Drawing for the job (mm, zero at the part's lowest x, y, z). A direction names the side the tool comes from. Round coordinates to 2 decimals unless told otherwise and drop trailing zeros. Write each loop counter-clockwise with the first axis right and the second up, starting at its lowest first coordinate (ties: lowest second). Pieces come first, ordered by that corner, then holes.
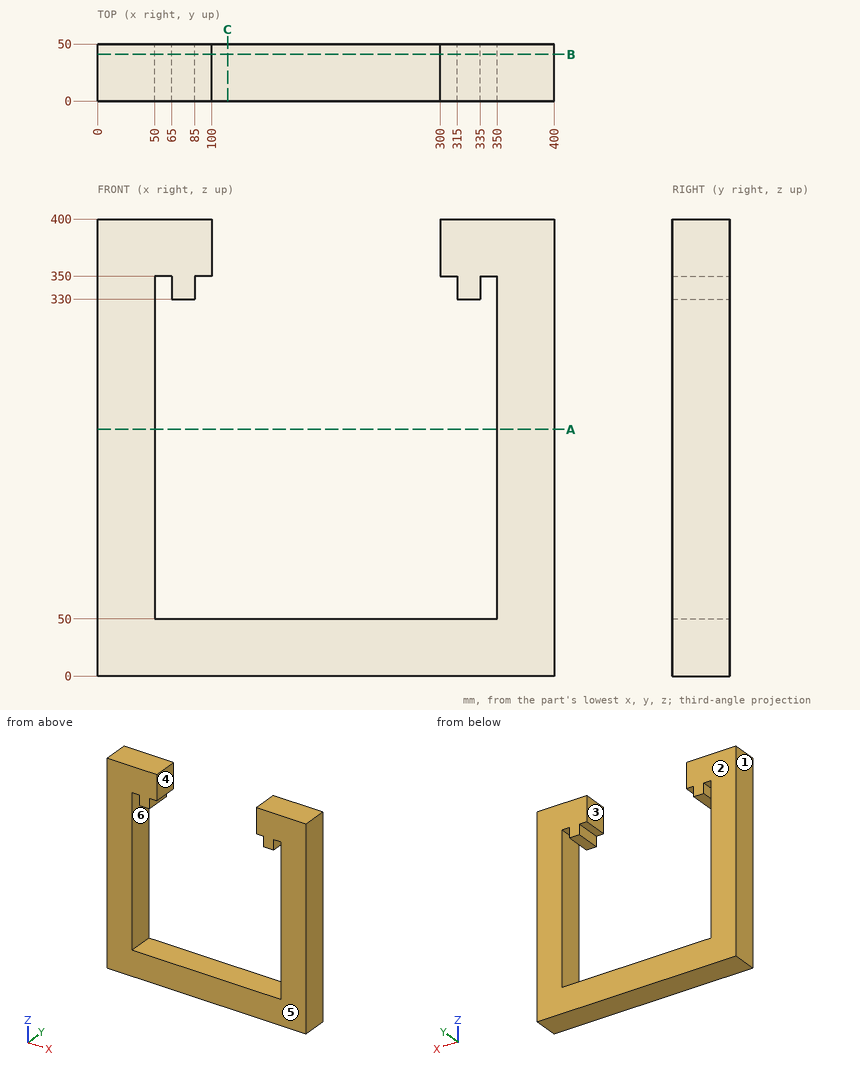
Q1. Saw through at B-B, the plane y = 41. Write the cut outline in (x, z), and give its area (3 significant figures).
Q2. Two-plate mould, pull along X, no slides. Class the marked faces 1, 2 and 3: released by +X, released by -X, zero draft, split by the parting line, or undercut.
Q3. Saw through at C-C, the plane x = 114. Write the cut outline in (y, z), and give its area (3 significant figures).
Q4. Tool access for the marked faces 4, 5 and 6: list every direction of +Z, -Z, +X, -X, +Y, -Y with a clear straight run to the whole face (end or side of a thin tool).
Q5. Drop a flat-ended pin along its axis: P1, Ø3, axis at x = 205.5, y = 26.5, coming from the +Z side. Give the stop position or say it passes through.
Q6. Saw through at A-A, the plane z = 216. Write the cut outline in (x, y).
Q7. Wall check: line 1 (X direction, y = 30.5, z = 182.5); line 2 (Z direction, x = 133, y = 31). Give the ranges that are in metal, low to high.
Computed:
1. outline: (0, 0) - (400, 0) - (400, 400) - (300, 400) - (300, 350) - (315, 350) - (315, 330) - (335, 330) - (335, 350) - (350, 350) - (350, 50) - (50, 50) - (50, 350) - (65, 350) - (65, 330) - (85, 330) - (85, 350) - (100, 350) - (100, 400) - (0, 400) - close
1. area: 60,800 mm2
2. face 1: released by -X
2. face 2: zero draft
2. face 3: undercut
3. outline: (0, 0) - (50, 0) - (50, 50) - (0, 50) - close
3. area: 2,500 mm2
4. face 4: +Z, +Y, -Y
4. face 5: +Z, -Z, +X, -X, -Y
4. face 6: +Y, -Y
5. P1: stops at z = 50
6. outline: (0, 0) - (50, 0) - (50, 50) - (0, 50) - close; (350, 0) - (400, 0) - (400, 50) - (350, 50) - close
7. line 1: x = 0 to 50, 350 to 400
7. line 2: z = 0 to 50
